```python
from build123d import *

# Parameters (mm, degrees)
BOSS_EXTRUDE1_DEPTH = 5
SKETCH2_W           = 70
SKETCH2_H           = 5
BOSS_EXTRUDE2_DEPTH = 10
SKETCH3_R           = 1.95
CUT_EXTRUDE1_DEPTH  = 45.158804332
FILLET1_R           = 10
SKETCH4_R           = 2.5
CUT_EXTRUDE2_DEPTH  = 63.84902545
SKETCH5_R           = 5
CUT_EXTRUDE3_DEPTH  = 17
FILLET2_R           = 5


with BuildPart() as part:
    # Sketch1 → Boss-Extrude1 (new body)
    with BuildSketch(Plane(origin=(0, 0, 0), x_dir=(1, 0, 0), z_dir=(0, 1, 0))):
        Polygon((-35, -25), (-20, -25), (20, -25), (35, -25), (35, -20), (20, -20), (20, 25), (-20, 25), (-20, -20), (-35, -20), align=None)
    extrude(amount=BOSS_EXTRUDE1_DEPTH)

    # Sketch2 → Boss-Extrude2 (add)
    with BuildSketch(Plane(origin=(0, 5, 0), x_dir=(1, 0, 0), z_dir=(0, 1, 0))):
        with Locations((0, -22.5)):
            Rectangle(SKETCH2_W, SKETCH2_H)
    extrude(amount=BOSS_EXTRUDE2_DEPTH)

    # Sketch3 → Cut-Extrude1 (cut, through all)
    with BuildSketch(Plane(origin=(0, 5, 0), x_dir=(1, 0, 0), z_dir=(0, 1, 0))):
        with Locations(Location((0, 12.5, 0), (0, 0, 270))):
            Circle(SKETCH3_R)
        with Locations(Location((0, -7.5, 0), (0, 0, 90))):
            Circle(SKETCH3_R)
        with Locations(Location((0, 2.5, 0), (0, 0, 270))):
            Circle(SKETCH3_R)
    extrude(amount=-CUT_EXTRUDE1_DEPTH, mode=Mode.SUBTRACT)

    # Fillet1
    fillet1_edges = [part.edges().sort_by_distance(p)[0] for p in [
        (-20, 2.5, 20),
        (20, 2.5, 20),
        (0, 5, 20),
    ]]
    fillet(fillet1_edges, radius=FILLET1_R - 0.0001)  # a hair under: the kernel refuses the full size

    # Sketch4 → Cut-Extrude2 (cut, through all)
    with BuildSketch(Plane.XY.offset(25)):
        with Locations((-27.5, 7.5)):
            Circle(SKETCH4_R)
        with Locations((27.5, 7.5)):
            Circle(SKETCH4_R)
    extrude(amount=-CUT_EXTRUDE2_DEPTH, mode=Mode.SUBTRACT)

    # Sketch5 → Cut-Extrude3 (cut)
    with BuildSketch(Plane(origin=(0, 0, 20), x_dir=(-1, 0, 0), z_dir=(0, 0, -1))):
        with Locations((27.5, 7.5)):
            Circle(SKETCH5_R)
        with Locations((-27.5, 7.5)):
            Circle(SKETCH5_R)
    extrude(amount=CUT_EXTRUDE3_DEPTH, mode=Mode.SUBTRACT)

    # Fillet2
    fillet2_edges = [part.edges().sort_by_distance(p)[0] for p in [
        (-20, 2.5, -25),
        (20, 2.5, -25),
    ]]
    fillet(fillet2_edges, radius=FILLET2_R)


solid = part.part
```
The model under review builds one solid part; all positions refer to its coordinate system, in mm. A direction names the side the tool comes from. Give positions to 0.01 mm unless a question says otherwise; leave off trailing zeros. Write each loop counter-clockwise with the first axis right and the second up, starting at its lowest first coordinate (ties: lowest second). Pieces come first, ordered by that corner, then holes. Notation, with made-up numbers: M 73,10.5 L 88,10.5 A24 ccw 88,49.5 Z; hole C -3,22.5 d3. An arc over 180 degrees is marked long. Write each question's results on one line, items separated by ' | '. Start each with the question number.
1. Insertion check: pin 1 Ø8 at (x, z) = (-19, -4.5) entering from +Y; pin 2 Ø8 at (y, z) = (8, -19) entering from -X; pin 3 Ø6.5 at (x, y) = (27.5, 7.5) entering from -Z; pin 4 Ø1 at (y, z) = (12.5, 17.5) entering from +X. Each pin has a flat end and moves straight along its axis. Give the tip position at first contact, or say it passes through.
2. Mouldability with a two-part tool opening along Z and no side actions: class faces 6 (the cylindrical face through (-0.75, 2.54, -0.7)), 7 (the flat face through (-35, 7, 23)), 8 (the cylindrical face through (-1.187, 2.535, -14.047)), 9 (the cylindrical face through (0.42, 8.01, 17.15)) as released by +Z, released by -Z, zero draft, split by the parting line, or undercut.
3. We need section B-B (y = 1.5). Write out the cut boundary in (x, z).
4. For faces 1 (the flat face through (-20, 2, -5)), 2 (the cylindrical face through (1.187, 2.535, 9.047)), 3 (the flat face through (20, 2, -5)), 4 (the flat face through (0, 15, 22)), 5 (the flat face through (-23, 8, 20)), list the 3-axis set-ups (+Z, -Z, +X, -X, +Y, -Y) from which the entire face can be reached by the end or side of a thin tool; tool diameter is ignored.
5. For probe 1 along X at (y, z) = (1.4, 7.5); probe 2 along Y at (x, z) = (-11.5, -18); probe 3 along Z at (x, y) = (-23, 7.75), list the stretches that pass through material, from the lowest coordinate up. Write a range as [from, to].
6. We need section A-A (z = -12.5). Write out the cut boundary in (x, y).
Results found:
1) pin 1: stops at y = 5 | pin 2: stops at x = -20 | pin 3: stops at z = 20 | pin 4: passes through
2) face 6: undercut | face 7: zero draft | face 8: undercut | face 9: released by -Z
3) outline: M -35,20 L -30,20 A10 cw -20,10 L -20,-20 A5 ccw -15,-25 L 15,-25 A5 ccw 20,-20 L 20,10 A10 cw 30,20 L 35,20 L 35,25 L -35,25 Z; hole C 0,-12.5 d3.9; hole C 0,-2.5 d3.9; hole C 0,7.5 d3.9
4) face 1: -Z, -X, +Y, -Y | face 2: +Y, -Y | face 3: -Z, +X, +Y, -Y | face 4: +Z, -Z, +X, -X, +Y | face 5: -Z
5) probe 1: x = [-20, -1.95], [1.95, 20] | probe 2: y = [0, 5] | probe 3: z = [20, 25]
6) outline: M -20,0 L -1.95,0 L -1.95,5 L -20,5 Z; M 1.95,0 L 20,0 L 20,5 L 1.95,5 Z
